```python
from build123d import *

# Parameters (mm, degrees)
EXTRUDE_1_DEPTH     = 60
SKETCH_2_W          = 34.498052415
SKETCH_2_H          = 50
CUT_EXTRUDE_1_DEPTH = 45
SKETCH_3_R          = 3
SKETCH_3_R_2        = 2.5
CUT_EXTRUDE_2_DEPTH = 91.816454432
SKETCH_6_R          = 2
CUT_EXTRUDE_3_DEPTH = 82.627431502


with BuildPart() as part:
    # 草图1 → 凸台-拉伸1 (new body)
    with BuildSketch(Plane.XY):
        Polygon((-11.342511753, -7.127659574), (-46.342511753, -7.127659574), (-46.342511753, 42.872340426), (-31.342511753, 42.872340426), align=None)
    extrude(amount=EXTRUDE_1_DEPTH)

    # 草图2 → 切除-拉伸1 (cut)
    with BuildSketch(Plane(origin=(0, 42.872340426, 0), x_dir=(1, 0, 0), z_dir=(0, 1, 0))):
        with Locations((-24.093485546, -30)):
            Rectangle(SKETCH_2_W, SKETCH_2_H)
    extrude(amount=-CUT_EXTRUDE_1_DEPTH, mode=Mode.SUBTRACT)

    # 草图3 → 切除-拉伸2 (cut, through all)
    with BuildSketch(Plane.XZ.offset(7.127659574)):
        with Locations((-35.342511753, 48)):
            Circle(SKETCH_3_R)
        with Locations(Location((-35.342511753, 12, 0), (0, 0, 270))):
            Circle(SKETCH_3_R)
        with Locations(Location((-19.342511753, 12, 0), (0, 0, 270))):
            Circle(SKETCH_3_R_2)
        with Locations((-19.342511753, 48)):
            Circle(SKETCH_3_R_2)
    extrude(amount=-CUT_EXTRUDE_2_DEPTH, mode=Mode.SUBTRACT)

    # 草图6 → 切除-拉伸3 (cut, through all)
    with BuildSketch(Plane.ZY.offset(46.342511753)):
        with Locations((53.5, 17.872340426)):
            Circle(SKETCH_6_R)
        with Locations(Location((6.5, 17.872340426, 0), (0, 0, 221.409622109))):
            Circle(SKETCH_6_R)
    extrude(amount=-CUT_EXTRUDE_3_DEPTH, mode=Mode.SUBTRACT)


solid = part.part
```
Work out the finished part from the listing and answer in its coordinate system (mm). A direction names the side the tool comes from. Give positions to 0.01 mm unless a question says otherwise; leave off trailing zeros. Order: outer loops, then holes, each group sorted by start corner. A loop starts at its lowest first (then second) coordinate and runs counter-clockwise, first axis right, second up.
1. The mould has two halves that part along Y. Classify faces 1 (the cylindrical face through (-38.27, -4.66, 12.65)), 2 (the flat face through (-42, 42.872, 30)), 3 (the cylindrical face through (-39.43, 17.11, 55.35)), 4 (the flat face through (-29, -7.128, 30)): released by +Y, released by -Y, zero draft, split by the parting line, or undercut.
Result sheet:
face 1: zero draft
face 2: released by +Y
face 3: undercut
face 4: released by -Y
2. Straight lines are drawn through the part: L1, parallel to Z at x = -19, y = 2.5; L2, parallel to X at y = -3.4, z = 12; L3, parallel to Y at x = -28.25, z = 53.5. For each, find the intervals that lie inside material, in ascending order.
Result sheet:
L1: z = 0 to 5, 55 to 60
L2: x = -46.34 to -38.34, -32.34 to -21.84, -16.84 to -12.83
L3: y = -7.13 to -2.13
3. Section A-A, the plane z = 6.5 is taken. Determine the outline of the cut face in (x, y).
Result sheet:
outline: (-46.34, -7.13) - (-11.34, -7.13) - (-13.34, -2.13) - (-41.34, -2.13) - (-41.34, 15.87) - (-46.34, 15.87) - close; (-46.34, 19.87) - (-41.34, 19.87) - (-41.34, 42.87) - (-46.34, 42.87) - close
4. Section C-C, the plane y = 9.5 is taken. Determine the outline of the cut face in (x, z).
Result sheet:
outline: (-46.34, 0) - (-17.99, 0) - (-17.99, 5) - (-41.34, 5) - (-41.34, 55) - (-17.99, 55) - (-17.99, 60) - (-46.34, 60) - close
5. Section D-D, the plane z = 27.5 is taken. Determine the outline of the cut face in (x, y).
Result sheet:
outline: (-46.34, -7.13) - (-11.34, -7.13) - (-13.34, -2.13) - (-41.34, -2.13) - (-41.34, 42.87) - (-46.34, 42.87) - close
6. Each of these flat-tipped pins is pushed along its axis until it touches: P1, Ø2, axis at x = -30, z = 6.5, coming from the +Y side; P2, Ø5, axis at y = -0.5, z = 21, coming from the +X side; P3, Ø4, axis at y = 18, z = 36, coming from the +X side. Where does it stop, or does it pass through?
Result sheet:
P1: stops at y = -2.13
P2: stops at x = -12.99
P3: stops at x = -41.34
7. Section B-B, the plane x = -33.5 is taken. Determine the outline of the cut face in (y, z).
Result sheet:
outline: (-7.13, 0) - (42.87, 0) - (42.87, 5) - (19.2, 5) arc R2 cw to (16.55, 5) - (-2.13, 5) - (-2.13, 9.63) - (-7.13, 9.63) - close; (-7.13, 14.37) - (-2.13, 14.37) - (-2.13, 45.63) - (-7.13, 45.63) - close; (-7.13, 50.37) - (-2.13, 50.37) - (-2.13, 55) - (16.55, 55) arc R2 cw to (19.2, 55) - (42.87, 55) - (42.87, 60) - (-7.13, 60) - close
8. For faces 5 (the flat face through (-28, -2.128, 30)), 6 (the cylindrical face through (-19.88, -4.66, 45.56)), determine the directions among +Z, -Z, +X, -X, +Y, -Y from which every point of the face is accessible in a straight line to the end or side of a thin tool.
Result sheet:
face 5: +X, +Y
face 6: +Y, -Y
